from build123d import *

# Parameters (mm, degrees)
F0_R     = 8.5
F1_DEPTH = 20
F2_R     = 4.6
F3_DEPTH = 4.8
F5_DEPTH = 12.5
F6_W     = 6.6
F6_H     = 6.6
F7_DEPTH = 7


with BuildPart() as f1:
    # F0 (on Top) → F1 (new body)
    with BuildSketch(Plane.XY):
        Circle(F0_R)
    extrude(amount=F1_DEPTH)

    # F2 (on face) → F3 (cut)
    with BuildSketch(Plane.XY.offset(20)):
        Circle(F2_R)
    extrude(amount=-F3_DEPTH, mode=Mode.SUBTRACT)

    # F4 (on Front) → F5 (cut, symmetric)
    with BuildSketch(Plane.XZ):
        with BuildLine():
            Line((-1.5, 20), (-1.5, 18.3))
            ThreePointArc((-1.5, 18.3), (0, 16.8), (1.5, 18.3))
            Line((1.5, 18.3), (1.5, 20))
            Line((1.5, 20), (-1.5, 20))
        make_face()
    extrude(amount=F5_DEPTH, both=True, mode=Mode.SUBTRACT)

    # F6 (on face) → F7 (cut)
    with BuildSketch(Plane(origin=(0, 0, 0), x_dir=(1, 0, 0), z_dir=(0, 0, -1))):
        Rectangle(F6_W, F6_H)
    extrude(amount=-F7_DEPTH, mode=Mode.SUBTRACT)


solid = f1.part
Could you check a few things on this model? Use its own coordinates, in mm. A direction names the side the tool comes from. Round coordinates to 2 decimals unless told otherwise and drop trailing zeros. Loops run counter-clockwise (first coordinate to the right, second up) from the corner with the lowest first, then second, coordinate; pieces in that order, holes last. Notation, with made-up numbers: (-15.5, -3) - (37.5, -3) arc R15 ccw to (37.5, 23) - close; hole circle Ø4 at (61, 67). An arc over 180 degrees is marked (long way). Write item = value, one per line.
1) I'm going to push flat-ended pins straight in: P1, Ø4, axis at y = -2, z = 6, coming from the +X side; P2, Ø3, axis at x = 1, y = 1.5, coming from the +Z side; P3, Ø3, axis at x = 3.5, z = 10, coming from the +Y side; P4, Ø5, axis at y = 4, z = 4.5, coming from the +X side. Where does each tip first touch, or does it pass through?
Computed:
P1 = 8.5
P2 = 15.2
P3 = 8.26
P4 = 8.37
2) Imagine slicing it at C-C (z = 6.25). Please give me the cut outline in (x, y).
Computed:
outline = circle Ø17 at (0, 0); hole (-3.3, -3.3) - (3.3, -3.3) - (3.3, 3.3) - (-3.3, 3.3) - close
3) If we mould it in two halves opening along X, with no side actions, what happens to faces 6 (the cylindrical face through (-1.84, -8.3, 9.86)), 7 (the cylindrical face through (0, -6.5, 16.8)), 8 (the flat face through (5, 0, 20))? For each: pulls with the +X half, pulls with the -X half, needs draft (parallel to the pull), parting line crosses it, or undercut.
Computed:
face_6 = parting line crosses it
face_7 = undercut
face_8 = needs draft
4) Imagine slicing it at B-B (y = 0). Please give me the cut outline in (x, z), and give its area (3 significant figures).
Computed:
outline = (-8.5, 0) - (-3.3, 0) - (-3.3, 7) - (3.3, 7) - (3.3, 0) - (8.5, 0) - (8.5, 20) - (4.6, 20) - (4.6, 15.2) - (-4.6, 15.2) - (-4.6, 20) - (-8.5, 20) - close
area = 250 mm2
5) Imagine slicing it at D-D (z = 13.25). Please give me the cut outline in (x, y).
Computed:
outline = circle Ø17 at (0, 0)
6) On a 3-axis mill with a long thin cutter (end or side, diameter ignored), from which of +Z, -Z, +X, -X, +Y, -Y can I reach the whole of each face in a straight line? I mean faces 1 (the flat face through (4, 0, 0)), 2 (the flat face through (-5, 0, 20)), 3 (the flat face through (3.3, 0, 3)), 4 (the cylindrical face through (4.25, -1.76, 17.63)), 5 (the flat face through (-1.5, -6, 19)). Say none if no direction works.
Computed:
face_1 = -Z, +X, -X, +Y, -Y
face_2 = +Z, +X, -X, +Y, -Y
face_3 = -Z
face_4 = +Z
face_5 = +Z, +Y, -Y
7) Imagine slicing it at A-A (x = 0). Please give me the cut outline in (y, z), and give its area (3 significant figures).
Computed:
outline = (-8.5, 0) - (-3.3, 0) - (-3.3, 7) - (3.3, 7) - (3.3, 0) - (8.5, 0) - (8.5, 16.8) - (4.6, 16.8) - (4.6, 15.2) - (-4.6, 15.2) - (-4.6, 16.8) - (-8.5, 16.8) - close
area = 225 mm2
8) I need wall thicknesses on line 1 along X through (y, z) = (0, 18.7); line 2 along X through (y, z) = (-1.5, 18); line 3 along Y through (x, z) = (-1.5, 1.75). Which ranges of each line are inside material? Lowest first, please. Write a range as from..to.
Computed:
line_1 = -8.5..-4.6, 4.6..8.5
line_2 = -8.37..-4.35, 4.35..8.37
line_3 = -8.37..-3.3, 3.3..8.37
